Geometry: final body of the model. Coordinates: model frame, mm. Give positions to 0.01 mm unless a question says otherwise; leave off trailing zeros. Write each loop counter-clockwise with the first axis right and the second up, starting at its lowest first coordinate (ties: lowest second). Pieces come first, ordered by that corner, then holes. Notation, with made-up numbers: (-21.5, 47) -> (-17.5, 47) arc R12 ccw to (-17.5, 66) -> close; hole circle Ø4 at (47.5, -37.5). An arc over 180 degrees is marked (long way). Answer in a Markdown table with one row per item. Add a question column.
Item 1: Material intervals for probe 1 along Y at (x, z) = (-50.5, 3.5); probe 2 along Y at (x, z) = (-128, 5.5); probe 3 along X at (y, z) = (79, 0.75), sorted ascending. Write a range as from..to.
Item 2: Section query B-B on x = -279.5. Output: boundary loops of the cut face in (y, z).
Item 3: First-contact query: P1, Ø6, axis at x = -88.5, y = 44.5, coming from the -Z side. Flat tip, straight axial feed; report the tip coordinate or a pass-through.
Item 4: Section query C-C on y = 24.5. State how many separate pieces and enclosed holes the cut face has, plus the area to 3 significant figures.
Item 5: Section query A-A on x = -118.5. Output: boundary loops of the cut face in (y, z).
```python
from build123d import *

# Parameters (mm, degrees)
MODEL_W             = 8.001
MODEL_H             = 8.001
BOSS_EXTRUDE1_DEPTH = 6.35


with BuildPart() as part:
    # Model → Boss-Extrude1 (new body)
    with BuildSketch(Plane.XY):
        Polygon((-398.78, 0), (-436.88, 63.5), (-436.88, 95.25), (0, 95.25), (0, 0), align=None)
        with Locations((-70.891200524, 88.9)):
            Rectangle(MODEL_W, MODEL_H, mode=Mode.SUBTRACT)
        Polygon((-235.938184475, 73.86541105), (-227.937630461, 73.78093355), (-227.853152962, 81.781487564), (-235.853706976, 81.865965064), align=None, mode=Mode.SUBTRACT)
        with BuildLine():
            Line((-171.232102448, 6.35), (-215.9, 6.35))
            ThreePointArc((-215.9, 6.35), (-220.390128061, 8.209871939), (-222.25, 12.7))
            Line((-222.25, 12.7), (-222.25, 57.367897552))
            ThreePointArc((-222.25, 57.367897552), (-220.682015918, 59.714551564), (-217.913948776, 59.163948776))
            Line((-217.913948776, 59.163948776), (-169.436051224, 10.686051224))
            ThreePointArc((-169.436051224, 10.686051224), (-168.885448436, 7.917984082), (-171.232102448, 6.35))
        make_face(mode=Mode.SUBTRACT)
        with BuildLine():
            Line((-234.95, 57.367897552), (-234.95, 12.7))
            ThreePointArc((-234.95, 12.7), (-236.809871939, 8.209871939), (-241.3, 6.35))
            Line((-241.3, 6.35), (-285.967897552, 6.35))
            ThreePointArc((-285.967897552, 6.35), (-288.314551564, 7.917984082), (-287.763948776, 10.686051224))
            Line((-287.763948776, 10.686051224), (-239.286051224, 59.163948776))
            ThreePointArc((-239.286051224, 59.163948776), (-236.517984082, 59.714551564), (-234.95, 57.367897552))
        make_face(mode=Mode.SUBTRACT)
        with BuildLine():
            Line((-294.113948776, 17.036051224), (-245.636051224, 65.513948776))
            ThreePointArc((-245.636051224, 65.513948776), (-245.085448436, 68.282015918), (-247.432102448, 69.85))
            Line((-247.432102448, 69.85), (-292.1, 69.85))
            ThreePointArc((-292.1, 69.85), (-296.590128061, 67.990128061), (-298.45, 63.5))
            Line((-298.45, 63.5), (-298.45, 18.832102448))
            ThreePointArc((-298.45, 18.832102448), (-296.882015918, 16.485448436), (-294.113948776, 17.036051224))
        make_face(mode=Mode.SUBTRACT)
        with BuildLine():
            Line((-323.632102448, 6.35), (-368.3, 6.35))
            ThreePointArc((-368.3, 6.35), (-372.790128061, 8.209871939), (-374.65, 12.7))
            Line((-374.65, 12.7), (-374.65, 57.367897552))
            ThreePointArc((-374.65, 57.367897552), (-373.082015918, 59.714551564), (-370.313948776, 59.163948776))
            Line((-370.313948776, 59.163948776), (-321.836051224, 10.686051224))
            ThreePointArc((-321.836051224, 10.686051224), (-321.285448436, 7.917984082), (-323.632102448, 6.35))
        make_face(mode=Mode.SUBTRACT)
        with BuildLine():
            Line((-18.832102448, 6.35), (-63.5, 6.35))
            ThreePointArc((-63.5, 6.35), (-67.990128061, 8.209871939), (-69.85, 12.7))
            Line((-69.85, 12.7), (-69.85, 57.367897552))
            ThreePointArc((-69.85, 57.367897552), (-68.282015918, 59.714551564), (-65.513948776, 59.163948776))
            Line((-65.513948776, 59.163948776), (-17.036051224, 10.686051224))
            ThreePointArc((-17.036051224, 10.686051224), (-16.485448436, 7.917984082), (-18.832102448, 6.35))
        make_face(mode=Mode.SUBTRACT)
        with BuildLine():
            Line((-82.55, 57.367897552), (-82.55, 12.7))
            ThreePointArc((-82.55, 12.7), (-84.409871939, 8.209871939), (-88.9, 6.35))
            Line((-88.9, 6.35), (-133.567897552, 6.35))
            ThreePointArc((-133.567897552, 6.35), (-135.914551564, 7.917984082), (-135.363948776, 10.686051224))
            Line((-135.363948776, 10.686051224), (-86.886051224, 59.163948776))
            ThreePointArc((-86.886051224, 59.163948776), (-84.117984082, 59.714551564), (-82.55, 57.367897552))
        make_face(mode=Mode.SUBTRACT)
        with BuildLine():
            Line((-93.236051224, 65.513948776), (-141.713948776, 17.036051224))
            ThreePointArc((-141.713948776, 17.036051224), (-144.482015918, 16.485448436), (-146.05, 18.832102448))
            Line((-146.05, 18.832102448), (-146.05, 63.5))
            ThreePointArc((-146.05, 63.5), (-144.190128061, 67.990128061), (-139.7, 69.85))
            Line((-139.7, 69.85), (-95.032102448, 69.85))
            ThreePointArc((-95.032102448, 69.85), (-92.685448436, 68.282015918), (-93.236051224, 65.513948776))
        make_face(mode=Mode.SUBTRACT)
        with BuildLine():
            Line((-163.086051224, 17.036051224), (-211.563948776, 65.513948776))
            ThreePointArc((-211.563948776, 65.513948776), (-212.114551564, 68.282015918), (-209.767897552, 69.85))
            Line((-209.767897552, 69.85), (-165.1, 69.85))
            ThreePointArc((-165.1, 69.85), (-160.609871939, 67.990128061), (-158.75, 63.5))
            Line((-158.75, 63.5), (-158.75, 18.832102448))
            ThreePointArc((-158.75, 18.832102448), (-160.317984082, 16.485448436), (-163.086051224, 17.036051224))
        make_face(mode=Mode.SUBTRACT)
        with BuildLine():
            Line((-315.486051224, 17.036051224), (-363.963948776, 65.513948776))
            ThreePointArc((-363.963948776, 65.513948776), (-364.514551564, 68.282015918), (-362.167897552, 69.85))
            Line((-362.167897552, 69.85), (-317.5, 69.85))
            ThreePointArc((-317.5, 69.85), (-313.009871939, 67.990128061), (-311.15, 63.5))
            Line((-311.15, 63.5), (-311.15, 18.832102448))
            ThreePointArc((-311.15, 18.832102448), (-312.717984082, 16.485448436), (-315.486051224, 17.036051224))
        make_face(mode=Mode.SUBTRACT)
        with BuildLine():
            Line((-6.35, 63.5), (-6.35, 18.832102448))
            ThreePointArc((-6.35, 18.832102448), (-7.917984082, 16.485448436), (-10.686051224, 17.036051224))
            Line((-10.686051224, 17.036051224), (-59.163948776, 65.513948776))
            ThreePointArc((-59.163948776, 65.513948776), (-59.714551564, 68.282015918), (-57.367897552, 69.85))
            Line((-57.367897552, 69.85), (-12.7, 69.85))
            ThreePointArc((-12.7, 69.85), (-8.209871939, 67.990128061), (-6.35, 63.5))
        make_face(mode=Mode.SUBTRACT)
    extrude(amount=BOSS_EXTRUDE1_DEPTH)


solid = part.part
```
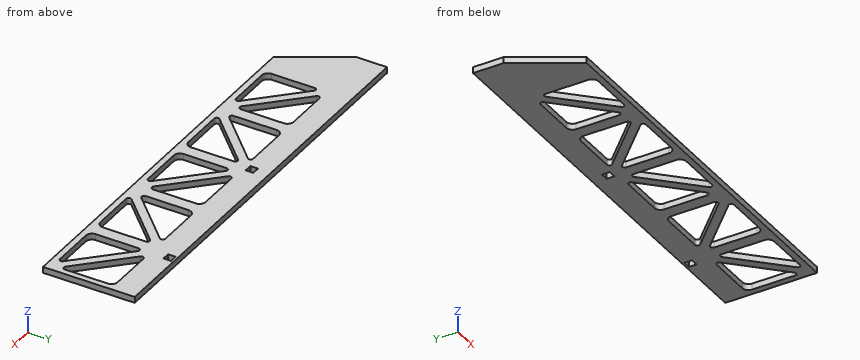
Findings below:
| question | item | result |
|---|---|---|
| 1 | probe 1 | y = 0..6.35, 44.15..56.85, 69.85..95.25 |
| 1 | probe 2 | y = 0..6.35, 18.05..30.75, 69.85..95.25 |
| 1 | probe 3 | x = -436.88..-235.88, -227.88..0 |
| 2 | outline | (0, 0) -> (6.35, 0) -> (6.35, 6.35) -> (0, 6.35) -> close; (18.95, 0) -> (31.65, 0) -> (31.65, 6.35) -> (18.95, 6.35) -> close; (69.85, 0) -> (95.25, 0) -> (95.25, 6.35) -> (69.85, 6.35) -> close |
| 3 | P1 | passes through |
| 4 | separate pieces | 11 |
| 4 | enclosed holes | 0 |
| 4 | area | 1,010 mm^2 |
| 5 | outline | (0, 0) -> (6.35, 0) -> (6.35, 6.35) -> (0, 6.35) -> close; (27.55, 0) -> (40.25, 0) -> (40.25, 6.35) -> (27.55, 6.35) -> close; (69.85, 0) -> (95.25, 0) -> (95.25, 6.35) -> (69.85, 6.35) -> close |
